Input: part model. Units: mm. Frame: model coordinates. Give positions to 0.01 mm unless a question says otherwise; leave off trailing zeros. Loops run counter-clockwise (first coordinate to the right, second up) from the corner with the lowest first, then second, coordinate; pieces in that order, holes last. Notation, with made-up numbers: (3, -28) -> (7, -28) arc R31 ccw to (7, 2) -> close; hole circle Ø7 at (70, -6). An arc over 180 degrees is marked (long way). Use CSV: the item, a comma, the result in double quotes.
```python
from build123d import *

# Parameters (mm, degrees)
EXTRUDE1_DEPTH     = 18.3
SKETCH2_R          = 3.01
CUT_EXTRUDE1_DEPTH = 15.5
FILLET1_R          = 2


with BuildPart() as part:
    # Sketch1 → Extrude1 (new body)
    with BuildSketch(Plane(origin=(0, 0, 0), x_dir=(0, 0, -1), z_dir=(1, 0, 0))):
        with BuildLine():
            Line((0, 0), (30, 0))
            Line((30, 0), (30, 26.2))
            ThreePointArc((30, 26.2), (15, 41.2), (0, 26.2))
            Line((0, 26.2), (0, 0))
        make_face()
    extrude(amount=EXTRUDE1_DEPTH)

    # Sketch2 → Cut-Extrude1 (cut)
    with BuildSketch(Plane.ZY):
        with Locations((-15, 26.2)):
            Circle(SKETCH2_R)
    extrude(amount=-CUT_EXTRUDE1_DEPTH, mode=Mode.SUBTRACT)

    # Fillet1
    fillet1_edges = [part.edges().sort_by_distance(p)[0] for p in [
        (18.3, 13.1, -30),
        (18.3, 41.2, -15),
        (18.3, 13.1, 0),
        (18.3, 0, -15),
        (9.15, 0, -30),
        (9.15, 0, 0),
    ]]
    fillet(fillet1_edges, radius=FILLET1_R)


solid = part.part
```
1) Contact query for flat-ended pins moving along their axis: pin 1 (2 mm diameter, centred on x = 3.5, z = -7, fed in from +Y); pin 2 (3 mm diameter, centred on x = 11.5, y = 32.5, fed in from -Z); pin 3 (3 mm diameter, centred on y = 27.5, z = -15, fed in from -X). Output: stop coordinate, or through.
From the geometry:
pin 1,"stops at y = 39.47"
pin 2,"stops at z = -29.21"
pin 3,"stops at x = 15.5"
2) Section query A-A (x = 5). Return loops of the section in (y, z), then the cut area to 3 significant figures.
From the geometry:
outline,"(0, -28) arc R2 ccw to (2, -30) -> (26.2, -30) arc R15 ccw to (26.2, 0) -> (2, 0) arc R2 ccw to (0, -2) -> close; hole circle Ø6.02 at (26.2, -15)"
area,"1,110 mm^2"
3) Mould query, pull axis Z, two halves, no side actions, for faces 1 (the cylindrical face through (17.7, 0.57, -15.18)), 2 (the cylindrical face through (7.642, 28.738, -13.382)), 3 (the flat face through (15.5, 26, -15)), 4 (the cylindrical face through (8.26, 0.57, -29.4)). Classes: pulls with the +Z half, pulls with the -Z half, needs draft (parallel to the pull), parting line crosses it, or undercut.
From the geometry:
face 1,"needs draft"
face 2,"undercut"
face 3,"undercut"
face 4,"pulls with the -Z half"
4) Section query C-C (y = 24). Return loops of the section in (x, z), then the cut area to 3 significant figures.
From the geometry:
outline,"(0, -30) -> (16.3, -30) arc R2 ccw to (18.3, -28) -> (18.3, -2) arc R2 ccw to (16.3, 0) -> (0, 0) -> (0, -12.95) -> (15.5, -12.95) -> (15.5, -17.05) -> (0, -17.05) -> close"
area,"484 mm^2"
5) Ray query, line 1 (Y direction, x = 9.25, z = -15); line 2 (Z direction, x = 6.5, y = 28); line 3 (Y direction, x = 16, z = -13.75). Return the intervals inside material, ascending.
From the geometry:
line 1,"y = 0 to 23.19, 29.21 to 41.2"
line 2,"z = -29.89 to -17.41, -12.59 to -0.11"
line 3,"y = 0 to 41.15"
6) Section query B-B (z = -15). Return loops of the section in (x, y), then the cut area to 3 significant figures.
From the geometry:
outline,"(0, 0) -> (16.3, 0) arc R2 ccw to (18.3, 2) -> (18.3, 39.2) arc R2 ccw to (16.3, 41.2) -> (0, 41.2) -> (0, 29.21) -> (15.5, 29.21) -> (15.5, 23.19) -> (0, 23.19) -> close"
area,"659 mm^2"
